Design review of the part shown in the three views and the two pictorial views. Dimensions are in mm from the part's minimum x, y and z. Coordinates: 2 decimals unless noted, no trailing zeros. Order: outer loops, then holes, each group sorted by start corner. A loop starts at its lowest first (then second) coordinate and runs counter-clockwise, first axis right, second up. Notation, with made-up numbers: (64, -9) -> (114, -9) arc R16 cw to (114, 10) -> close; hole circle Ø1 at (77, 66.25). An arc over 180 degrees is marked (long way). Write item = value, one per line. Start each with the question number.
1) Consider section A-A on y = 0.95. Give the boundary of the cut face in (x, z), and give its area (3 significant figures).
2) Wall thickness on probe 1 along X at (y, z) = (0.5, 0.1); probe 2 along Y at (x, z) = (2.75, 0.1); probe 3 along X at (y, z) = (2.5, 0.15): over which ranges is each line inside the solid? List them lowest first. Write a range as [from, to].
3) Consider section B-B on z = 0.05. Give the boundary of the cut face in (x, y), and give its area (3 significant figures).
4) Consider section C-C on y = 3. Give the boundary of the cut face in (x, z).
5) Consider section D-D on x = 4.5. Give the boundary of the cut face in (y, z), and give its area (3 significant figures).
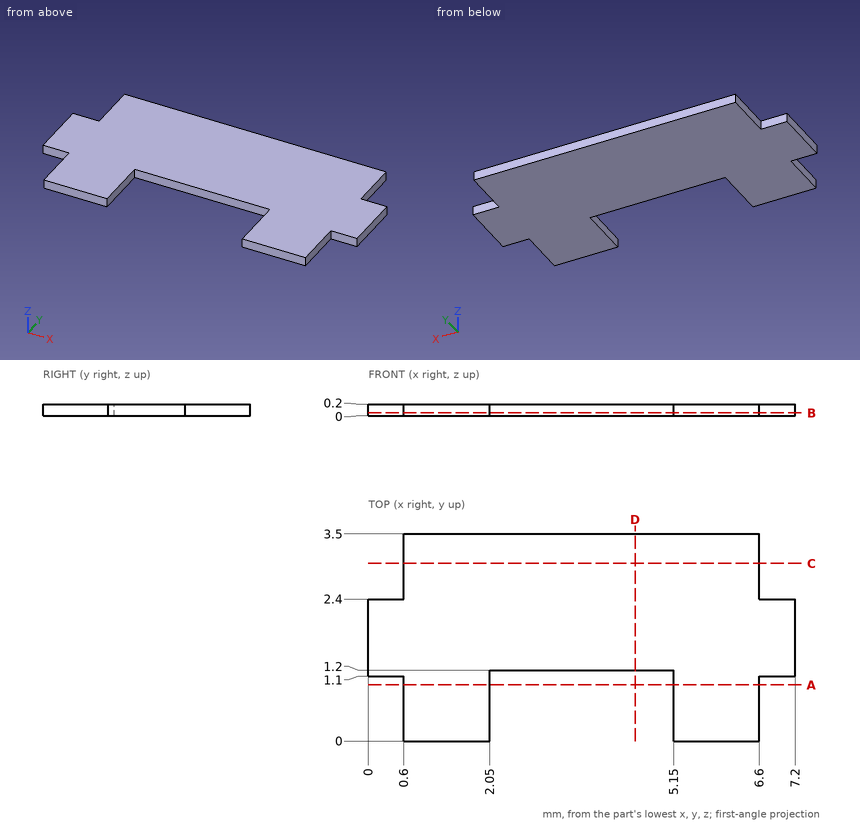
Answer sheet:
q1.outline = (0.6, 0) -> (2.05, 0) -> (2.05, 0.2) -> (0.6, 0.2) -> close; (5.15, 0) -> (6.6, 0) -> (6.6, 0.2) -> (5.15, 0.2) -> close
q1.area = 0.580 mm2
q2.probe_1 = [0.6, 2.05], [5.15, 6.6]
q2.probe_2 = [1.2, 3.5]
q2.probe_3 = [0.6, 6.6]
q3.outline = (0, 1.1) -> (0.6, 1.1) -> (0.6, 0) -> (2.05, 0) -> (2.05, 1.2) -> (5.15, 1.2) -> (5.15, 0) -> (6.6, 0) -> (6.6, 1.1) -> (7.2, 1.1) -> (7.2, 2.4) -> (6.6, 2.4) -> (6.6, 3.5) -> (0.6, 3.5) -> (0.6, 2.4) -> (0, 2.4) -> close
q3.area = 18.8 mm2
q4.outline = (0.6, 0) -> (6.6, 0) -> (6.6, 0.2) -> (0.6, 0.2) -> close
q5.outline = (1.2, 0) -> (3.5, 0) -> (3.5, 0.2) -> (1.2, 0.2) -> close
q5.area = 0.460 mm2
